from build123d import *

# Parameters (mm, degrees)
SALIENTE_EXTRUIR2_DEPTH = 0.4


with BuildPart() as part:
    # Croquis1 → Revolución1 (revolve)
    with BuildSketch(Plane.XY):
        Polygon((-10.9, 20), (-10.9, 0), (-12.25, 0), (-12.25, 18), (-22.25, 18), (-12.25, 20), align=None)
    revolve(axis=Axis((0, 0, 0), (0, 1, 0)))

    # Croquis3 → Saliente-Extruir2 (add)
    with BuildSketch(Plane(origin=(0, 20, 0), x_dir=(1, 0, 0), z_dir=(0, 1, 0))):
        with BuildLine():
            ThreePointArc((10.9, 0), (7.707463915, -7.707463915), (0, -10.9))
            ThreePointArc((0, -10.9), (-7.707463915, -7.707463915), (-10.9, 0))
            ThreePointArc((-10.9, 0), (-7.707463915, 7.707463915), (0, 10.9))
            ThreePointArc((0, 10.9), (7.707463915, 7.707463915), (10.9, 0))
        make_face()
        with BuildLine():
            Line((0.290070904, -3.989468495), (0, -10.639817501))
            Line((0, -10.639817501), (-0.290070904, -3.989468495))
            ThreePointArc((-0.290070904, -3.989468495), (-2.828427125, -2.828427125), (-3.989468495, -0.290070904))
            Line((-3.989468495, -0.290070904), (-10.639817501, 0))
            Line((-10.639817501, 0), (-3.989468495, 0.290070904))
            ThreePointArc((-3.989468495, 0.290070904), (-2.828427125, 2.828427125), (-0.290070904, 3.989468495))
            Line((-0.290070904, 3.989468495), (0, 10.639817501))
            Line((0, 10.639817501), (0.290070904, 3.989468495))
            ThreePointArc((0.290070904, 3.989468495), (2.828427125, 2.828427125), (3.989468495, 0.290070904))
            Line((3.989468495, 0.290070904), (10.639817501, 0))
            Line((10.639817501, 0), (3.989468495, -0.290070904))
            ThreePointArc((3.989468495, -0.290070904), (2.828427125, -2.828427125), (0.290070904, -3.989468495))
        make_face(mode=Mode.SUBTRACT)
    extrude(amount=-SALIENTE_EXTRUIR2_DEPTH)


solid = part.part
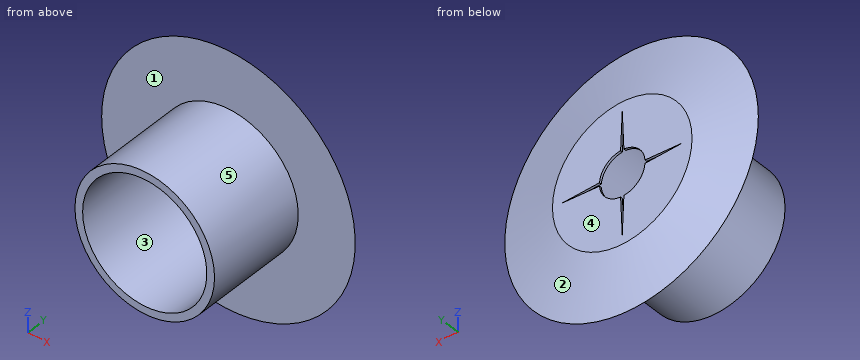
Read the model definition and answer for the solid it produces. Units are mm, in the model's axes. Face numbers are marked on the shaded views. A direction names the side the tool comes from. Give positions to 0.01 mm unless a question says otherwise; leave off trailing zeros. Write each loop counter-clockwise with the first axis right and the second up, starting at its lowest first coordinate (ties: lowest second). Pieces come first, ordered by that corner, then holes. Notation, with made-up numbers: (35, 70) - (56, 70) arc R12 cw to (56, 75) - close; hole circle Ø3 at (46, -6.75). An arc over 180 degrees is marked (long way). Return JSON: item names as keys, results as strings.
Q1. For a pull along X with two mould halves and no side action, classify the marked faces 1, 2 and 3 as released by +X, released by -X, zero draft, split by the parting line, or undercut.
Reply:
{"face 1": "zero draft", "face 2": "split by the parting line", "face 3": "undercut"}
Q2. Consider line 1 along Y through (x, z) = (-2, 8); line 2 along Z through (x, y) = (8.5, 14); line 3 along Z through (x, y) = (5, 5). Determine where each line is inside the solid, lowest interval first. Write a range as [from, to].
Reply:
{"line 1": "[19.6, 20]", "line 2": "[-8.82, -6.82], [6.82, 8.82]", "line 3": "[-11.18, -9.69], [9.69, 11.18]"}
Q3. Given P1, Ø1.5, axis at x = 13.5, z = 6, coming from the -Y side; P2, Ø5, axis at x = -10, z = 17, coming from the +Y side; P3, Ø6, axis at y = 4, z = 7, coming from the +X side, each flat-ended and moving along its own axis, determine where each tip first touches the part or whether it passes through.
Reply:
{"P1": "y = 18", "P2": "y = 19.01", "P3": "x = 11.58"}
Q4. For the marked faces 4 and 5, determine the directions among +Z, -Z, +X, -X, +Y, -Y from which every point of the face is accessible in a straight line to the end or side of a thin tool.
Reply:
{"face 4": "+Z, -Z, +X, -X, +Y", "face 5": "-Y"}
Q5. A cutting plane is placed at A-A, the plane y = 16. Determine the outline of the cut face in (x, z).
Reply:
{"outline": "circle Ø24.5 at (0, 0); hole circle Ø21.8 at (0, 0)"}
